The model under review builds one solid part; all positions refer to its coordinate system, in mm. A direction names the side the tool comes from. Coordinates: 2 decimals unless noted, no trailing zeros. Write each loop counter-clockwise with the first axis right and the second up, starting at its lowest first coordinate (ties: lowest second). Pieces come first, ordered by that corner, then holes. Notation, with made-up numbers: M 53,42 L 85,42 A10 ccw 85,61 Z; hole C 54,31.5 d6. An arc over 180 degrees is marked long. Answer as a JSON object with one key per item and string values.
```python
from build123d import *

# Parameters (mm, degrees)
F0_W      = 15
F0_H      = 5.08
F1_DEPTH  = 5.08
F1_FACE_W = 50
F1_FACE_H = 5.08
F2_DEPTH  = 25
F3_W      = 15
F3_H      = 5.08
F4_DEPTH  = 5.08
F5_W      = 15
F5_H      = 5.08
F6_DEPTH  = 5.08


with BuildPart() as f1:
    # F0 (on Front) → F1 (new body)
    with BuildSketch(Plane.XZ):
        Polygon((-87.5, 0), (0, 0), (0, 50), (-116.5, 50), (-144.902377, 50), (-196.5, 50), (-196.5, 101.597623), (-196.5, 130), (-246.5, 130), (-246.5, 0), (-231.5, 0), (-222.5, 0), (-207.5, 0), (-198.5, 0), (-183.5, 0), (-174.5, 0), (-159.5, 0), (-150.5, 0), (-135.5, 0), (-126.5, 0), (-111.5, 0), (-102.5, 0), align=None)
        Polygon((0, 50), (0, 0), (87.5, 0), (102.5, 0), (111.5, 0), (126.5, 0), (135.5, 0), (150.5, 0), (159.5, 0), (174.5, 0), (183.5, 0), (198.5, 0), (207.5, 0), (222.5, 0), (231.5, 0), (246.5, 0), (246.5, 130), (196.5, 130), (196.5, 101.597623), (196.5, 50), (144.902377, 50), (116.5, 50), align=None)
        with Locations((-95, -2.54)):
            Rectangle(F0_W, F0_H)
        with Locations((95, -2.54)):
            Rectangle(F0_W, F0_H)
        Polygon((-144.902377, 50), (-116.5, 50), (-196.5, 130), (-196.5, 101.597623), align=None)
        Polygon((196.5, 130), (116.5, 50), (144.902377, 50), (196.5, 101.597623), align=None)
        with Locations((-119, -2.54)):
            Rectangle(F0_W, F0_H)
        with Locations((119, -2.54)):
            Rectangle(F0_W, F0_H)
        with Locations((-143, -2.54)):
            Rectangle(F0_W, F0_H)
        with Locations((-239, -2.54)):
            Rectangle(F0_W, F0_H)
        with Locations((239, -2.54)):
            Rectangle(F0_W, F0_H)
        with Locations((143, -2.54)):
            Rectangle(F0_W, F0_H)
        with Locations((-167, -2.54)):
            Rectangle(F0_W, F0_H)
        with Locations((-215, -2.54)):
            Rectangle(F0_W, F0_H)
        with Locations((215, -2.54)):
            Rectangle(F0_W, F0_H)
        with Locations((167, -2.54)):
            Rectangle(F0_W, F0_H)
        with Locations((-191, -2.54)):
            Rectangle(F0_W, F0_H)
        with Locations((191, -2.54)):
            Rectangle(F0_W, F0_H)
    extrude(amount=F1_DEPTH)

    # F1_face (on face) → F2 (join)
    with BuildSketch(Plane(origin=(-221.5, -2.54, 130), x_dir=(1, 0, 0), z_dir=(0, 0, 1))):
        Rectangle(F1_FACE_W, F1_FACE_H)
        with Locations((443, 0)):
            Rectangle(F1_FACE_W, F1_FACE_H)
    extrude(amount=F2_DEPTH)

    # F3 (on face) → F4 (join)
    with BuildSketch(Plane.XY.offset(50)):
        with Locations((94, -2.54)):
            Rectangle(F3_W, F3_H)
    extrude(amount=F4_DEPTH)

    # F5 (on face) → F6 (join)
    with BuildSketch(Plane.XY.offset(50)):
        with Locations((-94, -2.54)):
            Rectangle(F5_W, F5_H)
    extrude(amount=F6_DEPTH)


solid = f1.part
```
(1) For pin 1 Ø2.5 at (x, y) = (-132, -1.5) entering from -Z, flat-tipped, find the tip position at first contact; note if it passes through.
Results list:
{"pin 1": "z = 0"}
(2) Add section A-A on z = 138. Give the boundary of the cut face in (x, y), and give its area (3 significant figures).
Results list:
{"outline": "M -246.5,-5.08 L -196.5,-5.08 L -196.5,0 L -246.5,0 Z; M 196.5,-5.08 L 246.5,-5.08 L 246.5,0 L 196.5,0 Z", "area": "508 mm²"}
(3) Add section B-B on z = 80. Give the boundary of the cut face in (x, y), and give its area (3 significant figures).
Results list:
{"outline": "M -246.5,-5.08 L -196.5,-5.08 L -196.5,0 L -246.5,0 Z; M -174.9,-5.08 L -146.5,-5.08 L -146.5,0 L -174.9,0 Z; M 146.5,-5.08 L 174.9,-5.08 L 174.9,0 L 146.5,0 Z; M 196.5,-5.08 L 246.5,-5.08 L 246.5,0 L 196.5,0 Z", "area": "797 mm²"}
(4) Add section D-D on z = 110. Give the boundary of the cut face in (x, y).
Results list:
{"outline": "M -246.5,-5.08 L -176.5,-5.08 L -176.5,0 L -246.5,0 Z; M 176.5,-5.08 L 246.5,-5.08 L 246.5,0 L 176.5,0 Z"}
(5) Add section C-C on y = -3.35. Count the separate pieces of the cut face and the enclosed holes in it, and give its area (3 significant figures).
Results list:
{"separate pieces": "1", "enclosed holes": "2", "area": "40,100 mm²"}
(6) Draft analysis for pull direction X (two halves, no side actions). For faces 4 (the face through (170.3, -2.5, 75.4)), 5 (the face through (-3, 0, 38)), 6 (the face through (157.1, -2.5, 90.6)), state which applies: released by +X, released by -X, zero draft, split by the parting line, or undercut.
Results list:
{"face 4": "undercut", "face 5": "zero draft", "face 6": "undercut"}
(7) Wall thickness on line 1 along X through (y, z) = (-4.05, 108); line 2 along Z through (x, y) = (2, -2); line 3 along X through (y, z) = (-0.4, 101): over which ranges is each line inside the solid? List them lowest first. Write a range as from..to.
Results list:
{"line 1": "-246.5..-174.5, 174.5..246.5", "line 2": "0..50", "line 3": "-246.5..-196.5, -195.9..-167.5, 167.5..195.9, 196.5..246.5"}
(8) For faces 1 (the face through (-3, -5.08, 38)), 2 (the face through (-155.9, -2.5, 89.4)), 3 (the face through (-171.1, -2.5, 76.2)), list the 3-axis set-ups (+Z, -Z, +X, -X, +Y, -Y) from which the entire face can be reached by the end or side of a thin tool; tool diameter is ignored.
Results list:
{"face 1": "+Z, -Z, +X, -X, -Y", "face 2": "+Z, +Y, -Y", "face 3": "+Y, -Y"}
